Source: CAD feature listing. Evaluate the final solid. Frame: model axes, mm. Face numbers are marked on the shaded views. A direction names the side the tool comes from. Give positions to 0.01 mm unless a question says otherwise; leave off trailing zeros. Loops run counter-clockwise (first coordinate to the right, second up) from the corner with the lowest first, then second, coordinate; pieces in that order, holes last. Notation, with made-up numbers: (69, 24.5) -> (121, 24.5) arc R25 cw to (121, 53.5) -> close; hole circle Ø9 at (-32, -30.75). An arc over 180 degrees is marked (long way). Return JSON: item names as keys, results as strings. Group by question number.
(1) Cut plane C-C on x = 21. Return loops of the section in (y, z).
(2) Pin query (flat end, axial travel): pin 1 (12 mm diameter, centred on x = 12, y = 4.5, fed in from -Z); pin 2 (9 mm diameter, centred on x = 20, y = 14, fed in from -Z); pin 3 (9 mm diameter, centred on x = 20, y = 14, fed in from +Z). Return the tip coordinate at first contact, or that it passes through.
(3) Draft query along Z for the marked faces 1, 2, 3 and 4. Return one class per face: released by +Z, released by -Z, zero draft, split by the parting line, or undercut.
(4) Access query for the marked faces 5, 6 and 7. Directions: +Z, -Z, +X, -X, +Y, -Y. A direction counts if a zero-diameter tool reaches every point of the face in a straight line with its end or side. Return the directions, or none.
(5) Cut plane D-D on x = -7. Return loops of the section in (y, z), then the cut area to 3 significant figures.
(6) Cut plane A-A on y = 17. Return loops of the section in (x, z).
(7) Cut plane B-B on z = 6. Return loops of the section in (x, y), then the cut area to 3 significant figures.
(8) Ray query, line 1 (X direction, y = 10.5, z = 5.5); line 2 (Z direction, x = 24.5, y = 14.75); line 3 (X direction, y = 3.5, z = -4.5). Return the intervals inside material, ascending. Write a range as from..to.
```python
from build123d import *

# Parameters (mm, degrees)
SKETCH1_R           = 7.5
BOSS_EXTRUDE1_DEPTH = 22
CUT_EXTRUDE1_REACH  = 41.9
SKETCH2_R           = 4


with BuildPart() as part:
    # Sketch1 → Boss-Extrude1 (new body)
    with BuildSketch(Plane(origin=(0, 0, 0), x_dir=(1, 0, 0), z_dir=(0, 1, 0))):
        with BuildLine():
            Line((28, 7.5), (7.348469228, 7.5))
            ThreePointArc((7.348469228, 7.5), (-10.5, 0), (7.348469228, -7.5))
            Line((7.348469228, -7.5), (28, -7.5))
            Line((28, -7.5), (28, -4))
            Line((28, -4), (12, -4))
            Line((12, -4), (12, 4))
            Line((12, 4), (28, 4))
            Line((28, 4), (28, 7.5))
        make_face()
        with Locations(Location((0, 0, 0), (0, 0, 270))):
            Circle(SKETCH1_R, mode=Mode.SUBTRACT)
    extrude(amount=BOSS_EXTRUDE1_DEPTH)

    # Cut-Extrude1: up to this face of the body (flat: up to its plane)
    cut_extrude1_end = Plane(part.part.faces().sort_by_distance((17.674234614, 11, -7.5))[0])
    # Sketch2 → Cut-Extrude1 (cut, up to the picked face)
    with BuildSketch(Plane.XY.offset(7.5), mode=Mode.PRIVATE) as cut_extrude1_sk1:
        with Locations((20, 14)):
            Circle(SKETCH2_R)
    cut_extrude1_tool1 = split(extrude(cut_extrude1_sk1.sketch, amount=-CUT_EXTRUDE1_REACH, mode=Mode.PRIVATE), bisect_by=cut_extrude1_end, keep=Keep.BOTH, mode=Mode.PRIVATE)
    # Sketch2 → Cut-Extrude1 (cut, up to the picked face)
    with BuildSketch(Plane.XY.offset(7.5), mode=Mode.PRIVATE) as cut_extrude1_sk2:
        Polygon((28, 9.077491087), (13.602007738, 0), (28, 0), align=None)
    cut_extrude1_tool2 = split(extrude(cut_extrude1_sk2.sketch, amount=-CUT_EXTRUDE1_REACH, mode=Mode.PRIVATE), bisect_by=cut_extrude1_end, keep=Keep.BOTH, mode=Mode.PRIVATE)
    # Sketch2 → Cut-Extrude1 (cut, up to the picked face)
    with BuildSketch(Plane.XY.offset(7.5), mode=Mode.PRIVATE) as cut_extrude1_sk3:
        with BuildLine():
            Line((20, 22), (20, 25.764527095))
            Line((20, 25.764527095), (29.423240249, 25.764527095))
            Line((29.423240249, 25.764527095), (29.423240249, 14))
            Line((29.423240249, 14), (28, 14))
            ThreePointArc((28, 14), (25.656854249, 19.656854249), (20, 22))
        make_face()
    cut_extrude1_tool3 = split(extrude(cut_extrude1_sk3.sketch, amount=-CUT_EXTRUDE1_REACH, mode=Mode.PRIVATE), bisect_by=cut_extrude1_end, keep=Keep.BOTH, mode=Mode.PRIVATE)
    add(cut_extrude1_tool1.solids().sort_by(Axis((20, 14, 7.5), (0, 0, -1)))[0], mode=Mode.SUBTRACT)
    add(cut_extrude1_tool2.solids().sort_by(Axis((23.200669, 3.02583, 7.5), (0, 0, -1)))[0], mode=Mode.SUBTRACT)
    add(cut_extrude1_tool3.solids().sort_by(Axis((25.803554, 21.945292, 7.5), (0, 0, -1)))[0], mode=Mode.SUBTRACT)


solid = part.part
```
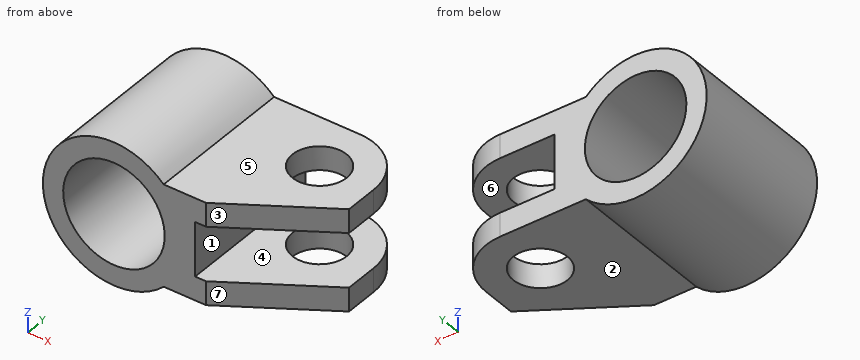
Answers:
{
 "1": {"outline": "(4.66, -7.5) -> (10.13, -7.5) -> (10.13, -4) -> (4.66, -4) -> close; (4.66, 4) -> (10.13, 4) -> (10.13, 7.5) -> (4.66, 7.5) -> close; (17.87, -7.5) -> (21.94, -7.5) -> (21.94, -4) -> (17.87, -4) -> close; (17.87, 4) -> (21.94, 4) -> (21.94, 7.5) -> (17.87, 7.5) -> close"},
 "2": {"pin 1": "z = -8.62", "pin 2": "z = -7.5", "pin 3": "z = 7.5"},
 "3": {"face 1": "undercut", "face 2": "released by -Z", "face 3": "zero draft", "face 4": "undercut"},
 "4": {"face 5": "+Z, +X, +Y, -Y", "face 6": "+X, +Y, -Y", "face 7": "+Z, -Z, +X, -Y"},
 "5": {"outline": "(0, -7.83) -> (22, -7.83) -> (22, -2.69) -> (0, -2.69) -> close; (0, 2.69) -> (22, 2.69) -> (22, 7.83) -> (0, 7.83) -> close", "area": "226 mm²"},
 "6": {"outline": "(7.35, -7.5) -> (17.35, -7.5) -> (17.35, -4) -> (12, -4) -> (12, 4) -> (17.35, 4) -> (17.35, 7.5) -> (7.35, 7.5) arc R10.5 ccw (long way) to start; (22.65, -7.5) -> (27.42, -7.5) -> (27.42, -4) -> (22.65, -4) -> close; (22.65, 4) -> (27.42, 4) -> (27.42, 7.5) -> (22.65, 7.5) -> close; hole circle Ø15 at (0, 0)"},
 "7": {"outline": "(-8.62, 0) -> (-4.5, 0) -> (-4.5, 22) -> (-8.62, 22) -> close; (4.5, 0) -> (13.6, 0) -> (28, 9.08) -> (28, 14) arc R8 ccw to (20, 22) -> (4.5, 22) -> close; hole circle Ø8 at (20, 14)", "area": "478 mm²"},
 "8": {"line 1": "-8.94..-5.1, 5.1..18.06, 21.94..28", "line 2": "-7.5..-4, 4..7.5", "line 3": "-9.49..-6, 6..19.15"}
}
